Autodesk Inventor part; units mm, degrees
ref_plane "YZ Plane" through (0, 0, 0) normal (1, 0, 0) x (0, 1, 0)
ref_plane "XZ Plane" through (0, 0, 0) normal (0, 1, 0) x (-1, 0, 0)
ref_plane "XY Plane" through (0, 0, 0) normal (0, 0, 1) x (1, 0, 0)
sketch "Schizzo1" plane through (0, 0, 0) normal (0, 1, 0) x (-1, 0, 0)
  line L0 (10.0009, -10.0148) -> (9.0009, -10.0148)
  line L1 (-10, 9) -> (-10, 10)
  line L2 (-10, 12) -> (-10, 10)
  line L3 (-10, -10.0148) -> (-9, -10.0148)
  line L4 (9.0009, -10.0148) -> (8.0009, -10.0148)
  line L5 (-9, -10.0148) -> (-8, -10.0148)
  line L6 (-10, 9) -> (-10, 8)
  line L7 (-10, -10.0148) -> (-10, -7.7324)
  circle A0 centre (-0.2724, -0.2591) radius 9.5
  line L8 (12.5009, -8.0148) -> (12.5009, -10.0148)
  line L9 (12.5009, -10.0148) -> (10.0009, -10.0148)
  line L10 (12.5009, 7.9852) -> (12.5009, 9.9852)
  line L11 (8, 12.5) -> (10, 12.5)
  line L12 (12.5009, 9.9852) -> (12.5009, 12.5)
  line L13 (12.5009, 12.5) -> (10, 12.5)
  line L14 (-8, 12.5) -> (-10, 12.5)
  line L15 (-10, 12.5) -> (-10, 12)
  line L16 (8.0009, -10.0148) -> (7.5009, -10.0148)
  line L17 (-8, -10.0148) -> (-7.5, -10.0148)
  circle A1 centre (-8.1016, -8.2148) radius 1
  circle A2 centre (8.0009, 7.5) radius 1
  line L18 (12.5009, -7.0148) -> (12.5009, -8.0148)
  line L19 (-7, 12.5) -> (-8, 12.5)
  line L20 (7.5009, -10.0148) -> (4.5009, -10.0148)
  line L21 (-7.5, -10.0148) -> (-4.5, -10.0148)
  line L22 (4.5009, -11.5148) -> (5.0009, -11.5148)
  line L23 (5.0009, -11.5148) -> (5.0009, -12.5148)
  line L24 (4.5009, -11.5148) -> (4.5009, -10.0148)
  line L25 (-4.5, -11.5148) -> (-5, -11.5148)
  line L26 (-5, -11.5148) -> (-5, -12.5148)
  line L27 (-5, -12.5148) -> (5.0009, -12.5148)
  line L28 (-4.5, -11.5148) -> (-4.5, -10.0148)
  line L29 (4.5009, 11.5) -> (5.0009, 11.5)
  line L30 (-4.5, 12.5) -> (-7, 12.5)
  line L31 (5.0009, 10) -> (-4.5, 10)
  line L32 (-4.5, 11.5) -> (-5.5, 11.5)
  line L33 (-5.5, 11.5) -> (-5.5, 10)
  line L34 (-5.5, 10) -> (-4.5, 10)
  line L35 (-4.5, 11.5) -> (-4.5, 12.5)
  line L36 (4.5009, 11.5) -> (4.5009, 12.5)
  line L37 (4.5009, 11.5) -> (5.5009, 11.5)
  line L38 (5.5009, 11.5) -> (5.5009, 10)
  line L39 (5.5009, 10) -> (5.0009, 10)
  line L40 (8, 12.5) -> (4.5009, 12.5)
  line L41 (-10, -10.0148) -> (-10, -4.0148)
  line L42 (-10, 7.5) -> (-10, 4.5)
  line L43 (-10, 4.5) -> (-11.5, 4.5)
  line L44 (-11.5, 4.5) -> (-11.5, 5)
  line L45 (-11.5, 5) -> (-12.5, 5)
  line L46 (-10, -4.0148) -> (-11.5, -4.0148)
  line L47 (-11.5, -4.0148) -> (-11.5, -4.5148)
  line L48 (-11.5, -4.5148) -> (-12.5, -4.5148)
  line L49 (-10, 7.5) -> (-10, 8)
  line L50 (-12.5, 5) -> (-12.5, -4.5148)
  line L51 (12.5009, 4.5) -> (11.5009, 4.5)
  line L52 (11.5009, 4.5) -> (11.5009, 5.5)
  line L53 (11.5009, 5.5) -> (10.0009, 5.5)
  line L54 (12.5009, 4.5) -> (12.5009, 7.9852)
  line L55 (12.5009, -4.0148) -> (11.5009, -4.0148)
  line L56 (12.5009, -4.0148) -> (12.5009, -7.0148)
  line L57 (11.5009, -4.0148) -> (11.5009, -5.0148)
  line L58 (11.5009, -5.0148) -> (10.0009, -5.0148)
  line L59 (10.0009, -5.0148) -> (10.0009, 5.5)
  point P0 (0, 0)
  dimension "d45" = 2
  dimension "d54" = 2
  dimension "d56" = 0.5
  dimension "d59" = 0.5
  dimension "d72" = 2
  dimension "d81" = 3
  dimension "d82" = 0.5
  dimension "d83" = 0.5
  dimension "d87" = 1
  dimension "d90" = 0.5
  dimension "d92" = 0.5
  dimension "d93" = 1
extrude "Estrusione6" add sketch "Schizzo1" along normal blind 2
properties part number "Maschio-femmina"
The listing builds one solid part. Answer for the finished solid, in the listing's coordinates (mm). A direction names the side the tool comes from. Round coordinates to 2 decimals unless told otherwise and drop trailing zeros. Write each loop counter-clockwise with the first axis right and the second up, starting at its lowest first coordinate (ties: lowest second). Pieces come first, ordered by that corner, then holes. Notation, with made-up numbers: M 1,79 L 38,79 A8 ccw 38,92 Z; hole C -14.75,-39 d5. An arc over 180 degrees is marked long. Write each question's results on one line, items separated by ' | '. Start each with the question number.
(1) Each of these flat-tipped pins is pushed along its axis until it touches: P1, Ø0.5, axis at x = 12, y = 1.5, coming from the -Z side; P2, Ø0.8, axis at y = 1, z = -10.5, coming from the -X side; P3, Ø1, axis at x = -6, y = 1, coming from the -Z side. Where does it stop, or does it pass through?
(2) For faces 1 (the flat face through (-4.501, 1, 12)), 2 (the flat face through (5, 1, -12)), 3 (the flat face through (0, 1, 10)), 4 (the flat face through (-12, 1, -4.015)), 5 (the flat face through (12, 1, 5)), determine the directions among +Z, -Z, +X, -X, +Y, -Y from which every point of the face is accessible in a straight line to the end or side of a thin tool.
(3) The part is cut by section C-C, the plane y = 1.4. Give the number of separate pieces and of enclosed holes in the cut face, and give its area (3 significant figures).
(4) The part is cut by section B-B, the plane z = 6. Write down the section's boundary in (x, y).
(5) The part is cut by section D-D, the plane x = 11. Write down the section's boundary in (y, z), and give its area (3 significant figures).
(6) Find the intervals of material crossed by line 1 (Z direction, x = -10.25, y = 0.35); line 2 (X direction, y = 0.2, z = -8.5); line 3 (Z direction, x = 8, y = 0.45), in increasing order.
(7) Determine the mould class of faces 6 (the flat face through (-11.501, 1, 5)), 7 (the flat face through (11, 1, -4.015)), 8 (the flat face through (12.5, 1, 0)), 9 (the flat face through (-4.501, 1, -11)) for opening direction X: +X half, -X half, draft (parallel to the pull), parting line (faces both ways), or undercut.
(8) The part is cut by section A-A, the plane x = 6. Write down the section's boundary in (y, z).
Worked answers:
1) P1: stops at z = -4.51 | P2: stops at x = -4.5 | P3: stops at z = -10.01
2) face 1: +Z, +Y, -Y | face 2: -Z, +X, +Y, -Y | face 3: +Y, -Y | face 4: -X, +Y, -Y | face 5: +Z, +X, +Y, -Y
3) separate pieces: 1 | enclosed holes: 3 | area: 213 mm²
4) outline: M -12.5,0 L -6.87,0 L -6.87,2 L -12.5,2 Z; M 7.42,0 L 10,0 L 10,2 L 7.42,2 Z
5) outline: M 0,-4.01 L 2,-4.01 L 2,4.5 L 0,4.5 Z | area: 17.0 mm²
6) line 1: z = -10.01 to -5.01, 5.5 to 12.5 | line 2: x = -12.5 to -4.45, 5 to 7.14, 9.06 to 10 | line 3: z = -10.01 to -9.21, -7.22 to -5.78, 5.27 to 12.5
7) face 6: undercut | face 7: undercut | face 8: +X half | face 9: -X half
8) outline: M 0,-10.01 L 2,-10.01 L 2,-7.84 L 0,-7.84 Z; M 0,7.32 L 2,7.32 L 2,12.5 L 0,12.5 Z
